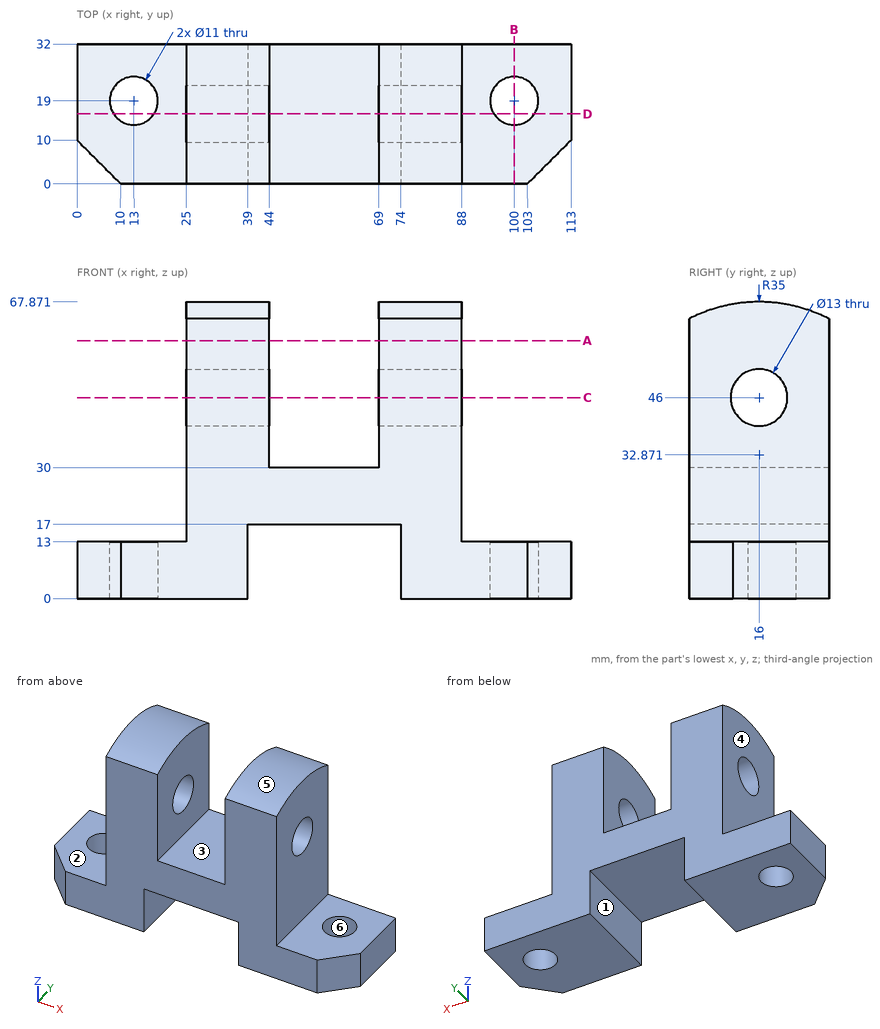
Print and shaded views of the part. All mm, measured from the part's lowest x, y and z. A direction names the side the tool comes from. Give positions to 0.01 mm unless a question says otherwise; leave off trailing zeros. Order: outer loops, then holes, each group sorted by start corner. A loop starts at its lowest first (then second) coordinate and runs counter-clockwise, first axis right, second up. Notation, with made-up numbers: M 82,15.5 L 126,15.5 A22 cw 126,25.5 Z; hole C 61.25,-33.5 d5. An arc over 180 degrees is marked long. Use one line per item in the form item = value.
Q1. Wall check: probe 1 along X at (y, z) = (4, 40); probe 2 along Y at (x, z) = (78.5, 46.5); probe 3 along X at (y, z) = (12, 6.5). Give the ranges that are in metal, low to high.
Conclusion:
probe_1 = 25 to 44, 69 to 88
probe_2 = 0 to 9.52, 22.48 to 32
probe_3 = 0 to 39, 74 to 113
Q2. Slice it at C-C, the plane z = 46. Write the cut outline in (x, y), and give its area (3 significant figures).
Conclusion:
outline = M 25,0 L 44,0 L 44,9.5 L 25,9.5 Z; M 25,22.5 L 44,22.5 L 44,32 L 25,32 Z; M 69,0 L 88,0 L 88,9.5 L 69,9.5 Z; M 69,22.5 L 88,22.5 L 88,32 L 69,32 Z
area = 722 mm2
Q3. Pin check, flat tips, straight feed: P1, Ø9.5, axis at y = 8, z = 57, coming from the +X side; P2, Ø5, axis at y = 26.5, z = 21, coming from the -X side; P3, Ø5, axis at x = 66.5, y = 13.5, coming from the -Z side; P4, Ø4, axis at x = 45.5, z = 33, coming from the -Y side. Stop position of each tip, or through.
Conclusion:
P1 = 88
P2 = 25
P3 = 17
P4 = 0
Q4. Pull direction X, two halves, no side cores. Call the marked faces 4, 5 and 6: released by +X, released by -X, zero draft, split by the parting line, or undercut.
Conclusion:
face_4 = released by -X
face_5 = zero draft
face_6 = undercut
Q5. Which spindle directions (+Z, -Z, +X, -X, +Y, -Y) get a long thin tool onto all of the face, cutting with end or side? Do the marked faces 1, 2 and 3. Say none if no direction does.
Conclusion:
face_1 = -Z, +Y, -Y
face_2 = +Z, -X, +Y, -Y
face_3 = +Z, +Y, -Y
Q6. Slice it at D-D, the plane y = 16. State how many separate pieces and enclosed holes the cut face has, and give its area (3 significant figures).
Conclusion:
separate_pieces = 5
enclosed_holes = 0
area = 2,650 mm2
Q7. Slice it at A-A, the plane z = 59. Write the cut outline in (x, y).
Conclusion:
outline = M 25,0 L 44,0 L 44,32 L 25,32 Z; M 69,0 L 88,0 L 88,32 L 69,32 Z
Q8. Slice it at B-B, the plane x = 100. Write the cut outline in (y, z), and give its area (3 significant figures).
Conclusion:
outline = M 0,0 L 13.5,0 L 13.5,13 L 0,13 Z; M 24.5,0 L 32,0 L 32,13 L 24.5,13 Z
area = 273 mm2
